```python
from build123d import *


with BuildPart() as f3:
    # F0 (on Front) → F3 section 0
    with BuildSketch(Plane.XZ, mode=Mode.PRIVATE) as f3_s0:
        Polygon((-56.9447709006, 57.9030166363), (-74.0163996816, 33.4221310914), (-81.0917035465, 4.4274015441), (-77.2151235029, -25.1652731148), (-62.9102131664, -51.359238194), (-40.1089299443, -70.6168535637), (-11.8907134819, -80.3372715581), (17.9334097249, -79.2076958644), (45.3355265759, -67.3806819392), (66.61482935, -46.4535335489), (78.8974302949, -19.2525780449), (80.5244960927, 10.5485448063), (71.2762824915, 38.9250282299), (52.4018119844, 62.0444709), (26.4501864003, 76.7844639748), (-3.0736834227, 81.1542897124), (-32.1824352676, 74.5637789329), align=None)
    loft([f3_s0.sketch, Vertex(0, -100, 9.4426637515)])


solid = f3.part
```
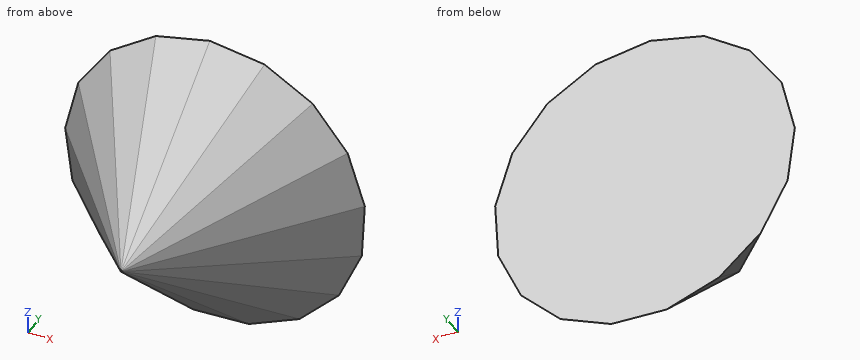
Read the model definition and answer for the solid it produces. Units are mm, in the model's axes. Give positions to 0.01 mm unless a question says otherwise; leave off trailing zeros. Order: outer loops, then holes, each group sorted by start corner. A loop starts at its lowest first (then second) coordinate and runs counter-clockwise, first axis right, second up. Notation, with made-up numbers: (39.25, 2.25) -> (68.25, 2.25) arc R25 ccw to (68.25, 40.25) -> close; hole circle Ø9 at (79.25, 6.5). An arc over 180 degrees is marked (long way). One line per item, written item: value. Start each with the question number.
(1) The part is cut by section A-A (z = -44). Determine the outline of the cut face in (x, y), and give its area (3 significant figures).
(2) Straight lines are drawn through the part: L1, parallel to Y at x = 30, z = -45; L2, parallel to Y at x = -58.5, z = 12; L3, parallel to Z at x = 5, y = -66. For each, find the intervals that lie inside material, in ascending order.
(3) The part is cut by section B-B (x = 41). Determine the outline of the cut face in (y, z), and give its area (3 significant figures).
(4) The part is cut by section C-C (y = -68.5). Determine the outline of the cut face in (x, z).
(5) The part is cut by section D-D (x = -50.5). Determine the outline of the cut face in (y, z).
(6) Flat-ended cylindrical pins translate along their axes: P1, Ø5, axis at y = -43, z = 55, coming from the -X side; P2, Ø10, axis at x = -22.5, y = -28.5, coming from the +Z side; P3, Ø2, axis at y = -26.5, z = -19, coming from the -X side; P4, Ø4, axis at x = 50, z = 50.5, coming from the -Y side. Find the tip coordinate at first contact, or state that the pin passes through.
Taken from the geometry:
1. outline: (-66.93, 0) -> (-55.3, -12.1) -> (-26.77, -33.25) -> (-7.08, -40.47) -> (10.81, -39.72) -> (31.54, -30.43) -> (63.69, -4.39) -> (67.72, 0) -> close
1. area: 3,460 mm^2
2. L1: -30.09 to 0
2. L2: -25.97 to 0
2. L3: -20.74 to 32.93
3. outline: (-49.08, 10.01) -> (-48.03, -5.47) -> (-38.45, -24.96) -> (-9.56, -60.03) -> (0, -69.25) -> (0, 68.52) -> (-21.76, 50.6) -> (-42.48, 26.4) -> close
3. area: 4,200 mm^2
4. outline: (-25.54, 7.86) -> (-24.32, -1.46) -> (-19.82, -9.71) -> (-12.63, -15.78) -> (-3.75, -18.84) -> (5.65, -18.48) -> (14.28, -14.76) -> (20.98, -8.16) -> (24.85, 0.4) -> (25.37, 9.79) -> (22.45, 18.73) -> (16.51, 26.01) -> (8.33, 30.66) -> (-0.97, 32.03) -> (-10.14, 29.96) -> (-17.94, 24.71) -> (-23.32, 17) -> close
5. outline: (-37.72, 6.32) -> (-34.6, -13.19) -> (-19.73, -39.36) -> (0, -61.84) -> (0, 62.24) -> (-11.32, 52.42) -> (-31.77, 25.8) -> close
6. P1: through
6. P2: z = 59.91
6. P3: x = -56.22
6. P4: y = -15.11
